```python
from build123d import *

# Parameters (mm, degrees)
SKETCH1_W               = 50
SKETCH1_H               = 50
SKETCH1_R               = 3.75
SKETCH1_R_2             = 2.75
BOSS_EXTRUDE1_DEPTH     = 3
BOSS_EXTRUDE2_DEPTH     = 50
CUT_EXTRUDE2_DEPTH      = 2
SKETCH10_W              = 50
SKETCH10_H              = 2.047418662
BOSS_EXTRUDE6_DEPTH     = 2
SKETCH11_W              = 5
SKETCH11_H              = 19
CUT_EXTRUDE4_DEPTH      = 4
SKETCH12_W              = 2
SKETCH12_H              = 50
BOSS_EXTRUDE7_DEPTH     = 10
SKETCH13_W              = 19
SKETCH13_H              = 5
CUT_EXTRUDE5_DEPTH      = 10
SKETCH14_R              = 5.75
SKETCH14_R_2            = 3.75
SKETCH14_R_3            = 4.75
SKETCH14_R_4            = 2.75
BOSS_EXTRUDE8_DEPTH     = 5
SKETCH15_W              = 50
SKETCH15_H              = 3
CUT_EXTRUDE6_DEPTH      = 161
CUT_EXTRUDE6_DEPTH_BACK = 15


with BuildPart() as part:
    # Sketch1 → Boss-Extrude1 (new body)
    with BuildSketch(Plane(origin=(0, 0, 0), x_dir=(1, 0, 0), z_dir=(0, 1, 0))):
        with Locations((0, 8.75)):
            Rectangle(SKETCH1_W, SKETCH1_H)
        Circle(SKETCH1_R, mode=Mode.SUBTRACT)
        with Locations((0, 17.5)):
            Circle(SKETCH1_R_2, mode=Mode.SUBTRACT)
    extrude(amount=BOSS_EXTRUDE1_DEPTH)

    # Sketch2 → Boss-Extrude2 (add)
    with BuildSketch(Plane.XY.offset(16.25)):
        Polygon((-25, 0), (-26.278653628, 0), (-74.233131713, 49.952581338), (-85, 49.952581338), (-85, 52), (-75, 52), (-75, 62), (-73, 62), (-73, 53), (-25, 3), align=None)
    boss_extrude2 = extrude(amount=-BOSS_EXTRUDE2_DEPTH)

    # Sketch3 → Cut-Extrude2 (cut)
    with BuildSketch(Plane(origin=(-11.511240633, -11.050791007, 0), x_dir=(0, 0, -1), z_dir=(0.721387321, 0.692531828, 0))):
        Polygon((-13.25, 85.788351472), (30.75, 85.788351472), (8.75, 25.788351472), align=None)
        Polygon((30.75, 77.073872213), (11.75, 25.255690395), (11.75, 19.477457668), (30.75, 19.477457668), (30.75, 22.897932802), align=None)
        Polygon((-13.25, 77.073872213), (-13.25, 19.477457668), (5.75, 19.477457668), (5.75, 25.255690395), align=None)
    cut_extrude2 = extrude(amount=-CUT_EXTRUDE2_DEPTH, mode=Mode.SUBTRACT)

    # Mirror1: Boss-Extrude2, Cut-Extrude2 across plane
    add(boss_extrude2.mirror(Plane(origin=(0, 0, 0), x_dir=(0, 0, 1), z_dir=(1, 0, 0))))
    add(cut_extrude2.mirror(Plane(origin=(0, 0, 0), x_dir=(0, 0, 1), z_dir=(1, 0, 0))), mode=Mode.SUBTRACT)

    # Sketch10 → Boss-Extrude6 (add)
    with BuildSketch(Plane(origin=(85, 0, 0), x_dir=(0, 0, -1), z_dir=(1, 0, 0))):
        with Locations((8.75, 50.976290669)):
            Rectangle(SKETCH10_W, SKETCH10_H)
    boss_extrude6 = extrude(amount=BOSS_EXTRUDE6_DEPTH)

    # Sketch11 → Cut-Extrude4 (cut)
    with BuildSketch(Plane(origin=(0, 49.952581338, 0), x_dir=(-1, 0, 0), z_dir=(0, -1, 0))):
        with Locations((-81.5, -3.75)):
            Rectangle(SKETCH11_W, SKETCH11_H)
        with Locations((-81.5, 21.25)):
            Rectangle(SKETCH11_W, SKETCH11_H)
    cut_extrude4 = extrude(amount=-CUT_EXTRUDE4_DEPTH, mode=Mode.SUBTRACT)

    # Mirror2: Boss-Extrude6, Cut-Extrude4 across plane
    add(boss_extrude6.mirror(Plane(origin=(0, 0, 0), x_dir=(0, 0, 1), z_dir=(1, 0, 0))))
    add(cut_extrude4.mirror(Plane(origin=(0, 0, 0), x_dir=(0, 0, 1), z_dir=(1, 0, 0))), mode=Mode.SUBTRACT)

    # Sketch12 → Boss-Extrude7 (add)
    with BuildSketch(Plane(origin=(0, 62, 0), x_dir=(1, 0, 0), z_dir=(0, 1, 0))):
        with Locations((74, 8.75)):
            Rectangle(SKETCH12_W, SKETCH12_H)
        with Locations((-74, 8.75)):
            Rectangle(SKETCH12_W, SKETCH12_H)
    extrude(amount=BOSS_EXTRUDE7_DEPTH)

    # Sketch13 → Cut-Extrude5 (cut)
    with BuildSketch(Plane.ZY.offset(-73)):
        with Locations((-21.25, 62.5)):
            Rectangle(SKETCH13_W, SKETCH13_H)
        with Locations((3.75, 62.5)):
            Rectangle(SKETCH13_W, SKETCH13_H)
    cut_extrude5 = extrude(amount=-CUT_EXTRUDE5_DEPTH, mode=Mode.SUBTRACT)

    # Mirror3: Cut-Extrude5 across plane
    add(cut_extrude5.mirror(Plane(origin=(0, 0, 0), x_dir=(0, 0, 1), z_dir=(1, 0, 0))), mode=Mode.SUBTRACT)

    # Sketch14 → Boss-Extrude8 (add)
    with BuildSketch(Plane(origin=(0, 3, 0), x_dir=(1, 0, 0), z_dir=(0, 1, 0))):
        Circle(SKETCH14_R)
        Circle(SKETCH14_R_2, mode=Mode.SUBTRACT)
        with Locations((0, 17.5)):
            Circle(SKETCH14_R_3)
        with Locations((0, 17.5)):
            Circle(SKETCH14_R_4, mode=Mode.SUBTRACT)
    extrude(amount=BOSS_EXTRUDE8_DEPTH)

    # Sketch15 → Cut-Extrude6 (cut, two sides)
    with BuildSketch(Plane.ZY.offset(-73)) as cut_extrude6_sk:
        with Locations((-8.75, 70.5)):
            Rectangle(SKETCH15_W, SKETCH15_H)
    extrude(amount=CUT_EXTRUDE6_DEPTH, mode=Mode.SUBTRACT)
    extrude(cut_extrude6_sk.sketch, amount=-CUT_EXTRUDE6_DEPTH_BACK, mode=Mode.SUBTRACT)


solid = part.part
```
Part model, mm, in its own coordinate system. A direction names the side the tool comes from. Round coordinates to 2 decimals unless told otherwise and drop trailing zeros. Write each loop counter-clockwise with the first axis right and the second up, starting at its lowest first coordinate (ties: lowest second). Pieces come first, ordered by that corner, then holes. Notation, with made-up numbers: M 65,8 L 70,8 A16 cw 70,35 Z; hole C 60,47.5 d9. An arc over 180 degrees is marked long. One line per question, with ' | ' between items.
(1) Saw through at C-C on x = 46. Write the cut outline in (y, z) (3 decimals).
Answer key:
outline: M 20.543,-33.75 L 24.875,-33.75 L 24.875,-30.75 L 21.987,-30.75 L 21.987,-19.986 L 24.875,-20.75 L 24.875,-17.555 L 21.987,-16.791 L 21.987,-0.709 L 24.875,0.055 L 24.875,3.25 L 21.987,2.486 L 21.987,13.25 L 24.875,13.25 L 24.875,16.25 L 20.543,16.25 Z
(2) Saw through at A-A on y = 57. Write the cut outline in (x, z), then the cut area to 3 significant figures.
Answer key:
outline: M -75,-33.75 L -73,-33.75 L -73,16.25 L -75,16.25 Z; M 73,-33.75 L 75,-33.75 L 75,16.25 L 73,16.25 Z | area: 200 mm^2
(3) Probe line 1 along Z through (x, y) = (0, 2); line 2 along X through (y, z) = (5, 0); line 3 along X through (y, z) = (3.5, 0). List the from-to ranges inside material, lowest first.
Answer key:
line 1: z = -33.75 to -20.25, -14.75 to -3.75, 3.75 to 16.25 | line 2: x = -31.08 to -29.69, -5.75 to -3.75, 3.75 to 5.75, 29.69 to 31.08 | line 3: x = -29.64 to -28.25, -5.75 to -3.75, 3.75 to 5.75, 28.25 to 29.64
(4) Two-plate mould, pull along Z, no slides. Class faces 1 (the face through (-3.746, 3.944, -0.165)), 2 (the face through (0, 1, 16.25)), 3 (the face through (-73, 61, -8)): released by +Z, released by -Z, zero draft, split by the parting line, or undercut.
Answer key:
face 1: undercut | face 2: released by +Z | face 3: zero draft
(5) Saw through at D-D on z = 0. Count the separate pieces of the cut face and the enclosed holes in it, then the cut area to 3 significant figures.
Answer key:
separate pieces: 6 | enclosed holes: 0 | area: 418 mm^2
(6) Saw through at B-B on x = 0. Write the cut outline in (y, z), then the cut area to 3 significant figures.
Answer key:
outline: M 0,-33.75 L 3,-33.75 L 3,-22.25 L 8,-22.25 L 8,-20.25 L 0,-20.25 Z; M 0,-14.75 L 8,-14.75 L 8,-12.75 L 3,-12.75 L 3,-5.75 L 8,-5.75 L 8,-3.75 L 0,-3.75 Z; M 0,3.75 L 8,3.75 L 8,5.75 L 3,5.75 L 3,16.25 L 0,16.25 Z | area: 151 mm^2
(7) 3-axis set-ups, long thin cutter, end or side, ignore diameter. For faces 4 (the face through (-81, 49.953, -8)), 5 (the face through (-81, 52, -8)), 6 (the face through (-47.405, 24.914, 3.617)), 7 (the face through (2, 8, -15)): which of +Z, -Z, +X, -X, +Y, -Y reach the whole face in a straight line?
Answer key:
face 4: +Z, -Z, -X, -Y | face 5: +Z, -Z, -X, +Y | face 6: none | face 7: +Z, -Z, +Y
(8) Pin check, flat tips, straight feed: pin 1 (4 mm diameter, centred on y = 41, z = -2.5, fed in from +X); pin 2 (4 mm diameter, centred on y = 24.5, z = -6, fed in from -X); pin 3 (1.5 mm diameter, centred on y = 48, z = -9, fed in from +X); pin 4 (8 mm diameter, centred on x = 58, y = 22, fed in from -Z). Stop position of each tip, or through.
Answer key:
pin 1: stops at x = 67.56 | pin 2: stops at x = -51.72 | pin 3: stops at x = 73.08 | pin 4: passes through
